from build123d import *

# Parameters (mm, degrees)
PAD_DEPTH            = 24.8
POCKET_DEPTH         = 24
SKETCH002_R          = 2.5
POCKET001_DEPTH      = 24.801
POCKET001_DEPTH_BACK = -0.001
POCKET002_DEPTH      = 188.754774
POCKET002_DEPTH_BACK = -163.954774
SKETCH004_W          = 4.5
SKETCH004_H          = 4.7
POCKET003_DEPTH      = 34.701
POCKET003_DEPTH_BACK = -34.701


with BuildPart() as part:
    # Sketch → Pad (new body)
    with BuildSketch(Plane.XY):
        with BuildLine():
            ThreePointArc((-15.95, 34.7), (-17.364214, 34.114214), (-17.95, 32.7))
            Line((-17.95, -32.7), (-17.95, 32.7))
            ThreePointArc((-17.95, -32.7), (-17.364214, -34.114214), (-15.95, -34.7))
            Line((15.95, -34.7), (-15.95, -34.7))
            ThreePointArc((15.95, -34.7), (17.364214, -34.114214), (17.95, -32.7))
            Line((17.95, 32.7), (17.95, -32.7))
            ThreePointArc((17.95, 32.7), (17.364214, 34.114214), (15.95, 34.7))
            Line((-15.95, 34.7), (15.95, 34.7))
        make_face()
    extrude(amount=-PAD_DEPTH)

    # Sketch001 → Pocket (cut)
    with BuildSketch(Plane.XY):
        with BuildLine():
            ThreePointArc((-15.55, 33.9), (-16.681371, 33.431371), (-17.15, 32.3))
            Line((-17.15, -32.3), (-17.15, 32.3))
            ThreePointArc((-17.15, -32.3), (-16.681371, -33.431371), (-15.55, -33.9))
            Line((15.55, -33.9), (-15.55, -33.9))
            ThreePointArc((15.55, -33.9), (16.681371, -33.431371), (17.15, -32.3))
            Line((17.15, 32.3), (17.15, -32.3))
            ThreePointArc((17.15, 32.3), (16.681371, 33.431371), (15.55, 33.9))
            Line((-15.55, 33.9), (15.55, 33.9))
        make_face()
    extrude(amount=-POCKET_DEPTH, mode=Mode.SUBTRACT)

    # Sketch002 → Pocket001 (cut, two sides)
    with BuildSketch(Plane.XY) as pocket001_sk:
        with Locations((10.9, -14.5)):
            Circle(SKETCH002_R)
        with Locations((-10.9, -14.5)):
            Circle(SKETCH002_R)
    extrude(amount=-POCKET001_DEPTH, mode=Mode.SUBTRACT)
    extrude(pocket001_sk.sketch, amount=-POCKET001_DEPTH_BACK, mode=Mode.SUBTRACT)

    # Sketch003 → Pocket002 (cut, two sides)
    with BuildSketch(Plane.XY) as pocket002_sk:
        with BuildLine():
            ThreePointArc((5, -8), (0, -3), (-5, -8))
            Line((-5, -8), (-5, -26))
            ThreePointArc((-5, -26), (0, -31), (5, -26))
            Line((5, -26), (5, -8))
        make_face()
    pocket002 = extrude(amount=-POCKET002_DEPTH, mode=Mode.SUBTRACT)
    extrude(pocket002_sk.sketch, amount=-POCKET002_DEPTH_BACK, mode=Mode.SUBTRACT)

    # Mirrored: Pocket002 across Sketch003 H_Axis
    add(pocket002.mirror(Plane.ZX), mode=Mode.SUBTRACT)

    # Sketch004 → Pocket003 (cut, two sides)
    with BuildSketch(Plane.XZ) as pocket003_sk:
        with Locations((0, -7.25)):
            Rectangle(SKETCH004_W, SKETCH004_H)
    extrude(amount=-POCKET003_DEPTH, mode=Mode.SUBTRACT)
    extrude(pocket003_sk.sketch, amount=-POCKET003_DEPTH_BACK, mode=Mode.SUBTRACT)


solid = part.part
Geometry check sheet. Reference: the model listing, model coordinates, mm. A direction names the side the tool comes from. Give positions to 0.01 mm unless a question says otherwise; leave off trailing zeros. Loops run counter-clockwise (first coordinate to the right, second up) from the corner with the lowest first, then second, coordinate; pieces in that order, holes last.
(1) Section check A-A on y = 12.5. Record the cut outline in (x, z), then the cut area to 3 significant figures.
From the geometry:
outline: (-17.95, -24.8) - (-5, -24.8) - (-5, -24) - (-17.15, -24) - (-17.15, 0) - (-17.95, 0) - close; (5, -24.8) - (17.95, -24.8) - (17.95, 0) - (17.15, 0) - (17.15, -24) - (5, -24) - close
area: 59.1 mm2
(2) Section check C-C on z = -6.25. Record the cut outline in (x, y).
From the geometry:
outline: (-17.95, -32.7) arc R2 ccw to (-15.95, -34.7) - (-2.25, -34.7) - (-2.25, -33.9) - (-15.55, -33.9) arc R1.6 cw to (-17.15, -32.3) - (-17.15, 32.3) arc R1.6 cw to (-15.55, 33.9) - (-2.25, 33.9) - (-2.25, 34.7) - (-15.95, 34.7) arc R2 ccw to (-17.95, 32.7) - close; (2.25, -34.7) - (15.95, -34.7) arc R2 ccw to (17.95, -32.7) - (17.95, 32.7) arc R2 ccw to (15.95, 34.7) - (2.25, 34.7) - (2.25, 33.9) - (15.55, 33.9) arc R1.6 cw to (17.15, 32.3) - (17.15, -32.3) arc R1.6 cw to (15.55, -33.9) - (2.25, -33.9) - close
(3) Set-up check for faces 1 (the cylindrical face through (-17.35, 34.13, -12.23)), 2 (the cylindrical face through (-0.1, -31, -24.4)), 3 (the flat face through (0, 33.9, -12)): record each of +Z, -Z, +X, -X, +Y, -Y from which the full face is reachable in a straight line by a thin tool's end or side.
From the geometry:
face 1: +Z, -Z, -X, +Y
face 2: +Z, -Z
face 3: +Z
(4) Section check D-D on x = 10.9. Record the cut outline in (y, z).
From the geometry:
outline: (-34.7, -24.8) - (-17, -24.8) - (-17, -24) - (-33.9, -24) - (-33.9, 0) - (-34.7, 0) - close; (-12, -24.8) - (34.7, -24.8) - (34.7, 0) - (33.9, 0) - (33.9, -24) - (-12, -24) - close
(5) Depth check by flat-ended pin: pin 1 Ø0.6 at (y, z) = (-34.5, -7.5) entering from +X; pin 2 Ø1.5 at (x, y) = (7, 1.5) entering from +Z; pin 3 Ø0.9 at (y, z) = (-34.5, -7) entering from -X. Enter the tip coordinate at first touch or a pass-through.
From the geometry:
pin 1: stops at x = 17.27
pin 2: stops at z = -24
pin 3: stops at x = -17.43
(6) Thickness scan on L1, parallel to Y at x = 10.9, z = -24.4; L2, parallel to X at y = -2.5, z = -4.5; L3, parallel to Y at x = 5.5, z = -14.5. Record the ranges inside material, lowest first.
From the geometry:
L1: y = -34.7 to -17, -12 to 34.7
L2: x = -17.95 to -17.15, 17.15 to 17.95
L3: y = -34.7 to -33.9, 33.9 to 34.7
(7) Section check B-B on y = -14.5. Record the cut outline in (x, z).
From the geometry:
outline: (-17.95, -24.8) - (-13.4, -24.8) - (-13.4, -24) - (-17.15, -24) - (-17.15, 0) - (-17.95, 0) - close; (-8.4, -24.8) - (-5, -24.8) - (-5, -24) - (-8.4, -24) - close; (5, -24.8) - (8.4, -24.8) - (8.4, -24) - (5, -24) - close; (13.4, -24.8) - (17.95, -24.8) - (17.95, 0) - (17.15, 0) - (17.15, -24) - (13.4, -24) - close
(8) Release check for a two-part mould opening along Y. For faces 4 (the flat face through (17.95, 0, -12)), 5 (the cylindrical face through (17.38, 34.1, -12.23)), 6 (the flat face through (0, -34.7, -12)), 7 (the cylindrical face through (16.67, -33.44, -11.83)) record: released by +Y, released by -Y, zero draft, split by the parting line, or undercut.
From the geometry:
face 4: zero draft
face 5: released by +Y
face 6: released by -Y
face 7: undercut
